Build history of the part. All positions in model axes, mm. Face numbers are marked on the shaded views. A direction names the side the tool comes from. Round coordinates to 2 decimals unless told otherwise and drop trailing zeros. Write each loop counter-clockwise with the first axis right and the second up, starting at its lowest first coordinate (ties: lowest second). Pieces come first, ordered by that corner, then holes. Notation, with made-up numbers: (-40, 86.25) - (16, 86.25) arc R19 cw to (16, 93.25) - close; hole circle Ø6 at (76, -22.75). An arc over 180 degrees is marked (long way). Answer as a JSON object with one key per item and string values. Group by question number.
Item 1: Slice it at D-D, the plane z = 3.25. List the corners of the cut face in (x, y), then the cut area to 3 significant figures.
Item 2: Slice it at B-B, the plane y = 0.75. List the corners of the cut face in (x, z), then the cut area to 3 significant figures.
Item 3: Which spindle directions (+Z, -Z, +X, -X, +Y, -Y) get a long thin tool onto all of the face, cutting with end or side? Do the marked faces 1, 2 and 3. Say none if no direction does.
Item 4: Flat gauge pins, fed straight in: pin 1 (1.2 mm diameter, centred on x = -9.5, z = 7, fed in from -Y); pin 2 (0.6 mm diameter, centred on y = -7.5, z = 4.5, fed in from -X); pin 3 (3 mm diameter, centred on x = 9, z = 4, fed in from +Y); pin 4 (0.5 mm diameter, centred on y = 9, z = 5, fed in from +X). Where does each tip first touch, or does it go through?
Item 5: Probe line 1 (X direction, y = -3.25, z = 5.75); line 2 (Y direction, x = -6, z = 4.25); line 3 (Y direction, x = -8.75, z = 4). List the from-to ranges inside material, lowest first. Write a range as from..to.
Item 6: Slice it at A-A, the plane x = 0. List the corners of the cut face in (y, z).
Item 7: Two-plate mould, pull along Y, no slides. Class the marked faces 4, 5 and 6: +Y half, -Y half, draft (parallel to the pull), parting line (faces both ways), or undercut.
Item 8: Slice it at C-C, the plane x = 5.5. List the corners of the cut face in (y, z).
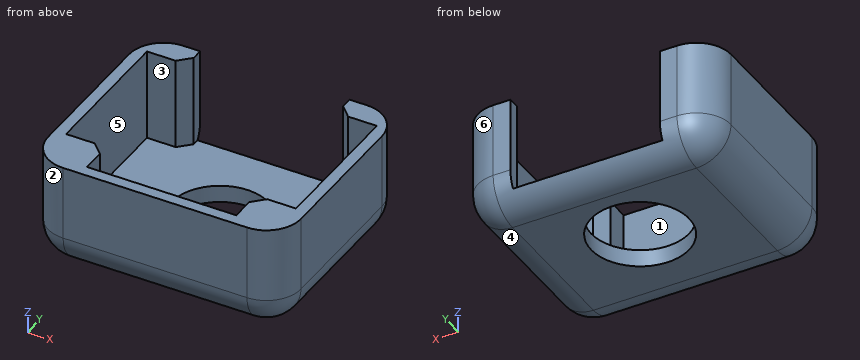
Solid Edge part; units mm, degrees
sketch "Sketch1" plane through (0, 0, 0) normal (0, 0, 1) x (1, 0, 0)
  line L0 (-11, -9.25) -> (11, -9.25)
  line L1 (11, -9.25) -> (11, 9.25)
  line L2 (11, 9.25) -> (-11, 9.25)
  line L3 (-11, 9.25) -> (-11, -9.25)
  circle A0 centre (0, 0.75) radius 4.25
  dimension "D1" = 11
  dimension "D2" = 11
extrude "Protrusion1" add sketch "Sketch1" along normal blind 1.5
sketch "Sketch2" plane through (0, 0, 1.5) normal (0, 0, 1) x (1, 0, 0)
  line L0 (11, -9.25) -> (6, -9.25)
  line L1 (6, -9.25) -> (6, -4.75)
  line L2 (6, -4.75) -> (11, -4.75)
  line L3 (11, -4.75) -> (11, -9.25)
  line L4 (-11, -9.25) -> (-6, -9.25)
  line L5 (-6, -9.25) -> (-6, -4.75)
  line L6 (-6, -4.75) -> (-11, -4.75)
  line L7 (-11, -4.75) -> (-11, -9.25)
  dimension "D1" = 11
  dimension "D2" = 11
  dimension "D3" = 11
  dimension "D4" = 11
extrude "bottom_extension" add sketch "Sketch2" along normal blind 8
sketch "Sketch3" plane through (0, 0, 1.5) normal (0, 0, 1) x (1, 0, 0)
  line L0 (-6, -9.25) -> (6, -9.25)
  line L1 (6, -9.25) -> (6, -8.25)
  line L2 (6, -8.25) -> (-6, -8.25)
  line L3 (-6, -8.25) -> (-6, -9.25)
  dimension "D1" = 6
extrude "Protrusion2" add sketch "Sketch3" along normal up to vertex (8 mm away)
sketch "Sketch4" plane through (0, 0.5, 1.5) normal (0, 0, 1) x (1, 0, 0)
  line L0 (11, 8.75) -> (6, 8.75)
  line L1 (6, 8.75) -> (6, 6.75)
  line L2 (6, 6.75) -> (11, 6.75)
  line L3 (11, 6.75) -> (11, 8.75)
  line L4 (-11, 8.75) -> (-6, 8.75)
  line L5 (-6, 8.75) -> (-6, 6.75)
  line L6 (-6, 6.75) -> (-11, 6.75)
  line L7 (-11, 6.75) -> (-11, 8.75)
  dimension "D1" = 11
  dimension "D2" = 11
extrude "Protrusion3" add sketch "Sketch4" along normal up to vertex (8 mm away)
sketch "Sketch5" plane through (0, 0.5, 1.5) normal (0, 0, 1) x (1, 0, 0)
  line L0 (-11, 6.75) -> (-10, 6.75)
  line L1 (-10, 6.75) -> (-10, -5.25)
  line L2 (-10, -5.25) -> (-11, -5.25)
  line L3 (-11, -5.25) -> (-11, 6.75)
  line L4 (11, -5.25) -> (10, -5.25)
  line L5 (10, -5.25) -> (10, 6.75)
  line L6 (10, 6.75) -> (11, 6.75)
  line L7 (11, 6.75) -> (11, -5.25)
  dimension "D1" = 11
  dimension "D2" = 11
extrude "Protrusion4" add sketch "Sketch5" along normal up to vertex (8 mm away)
fillet "Verrundung_1" radius 3 4 edges at (-11, 9.25, 4.75) (11, 9.25, 4.75) (11, -9.25, 4.75) (-11, -9.25, 4.75)
fillet "Verrundung_2" radius 3 7 edges at (0, -9.25, 0) (10.1213, -8.3713, 0) (11, 0, 0) (0, 9.25, 0) (-10.1213, 8.3713, 0) (-11, 0, 0) (-10.1213, -8.3713, 0)
sketch "Sketch6" plane through (0, 0, 9.5) normal (0, 0, 1) x (1, 0, 0)
  line L0 (-6, 9.25) -> (-6.5, 9.25)
  line L1 (-6.5, 9.25) -> (-6.5, 7.25)
  line L2 (-6.5, 7.25) -> (-6, 7.25)
  line L3 (-6, 7.25) -> (-6, 9.25)
  line L4 (6, 9.25) -> (6.5, 9.25)
  line L5 (6.5, 9.25) -> (6.5, 7.25)
  line L6 (6.5, 7.25) -> (6, 7.25)
  line L7 (6, 7.25) -> (6, 9.25)
  line L8 (-10, -4.75) -> (-6, -4.75)
  line L9 (-6, -4.75) -> (-6, -8.25)
  line L10 (-6.5, -8.25) -> (-6, -8.25)
  line L11 (-6.5, -5.25) -> (-6.5, -8.25)
  line L12 (-10, -5.25) -> (-6.5, -5.25)
  line L13 (-10, -5.25) -> (-10, -4.75)
  line L14 (6, -4.75) -> (10, -4.75)
  line L15 (10, -4.75) -> (10, -5.25)
  line L16 (10, -5.25) -> (6.5, -5.25)
  line L17 (6.5, -5.25) -> (6.5, -8.25)
  line L18 (6.5, -8.25) -> (6, -8.25)
  line L19 (6, -8.25) -> (6, -4.75)
  dimension "D1" = 6
extrude "Cutout1" cut sketch "Sketch6" against normal up to vertex (8 mm away)
chamfer "Fase_2" distance 1 angle 45 4 edges at (-6.5, 7.25, 5.5) (6.5, 7.25, 5.5) (6.5, -5.25, 5.5) (-6.5, -5.25, 5.5)
properties material "ABS-Plastik, mittelfest"
Geometry says:
{
 "1": {"outline": "(-11, -6.25) arc R3 ccw to (-8, -9.25) - (8, -9.25) arc R3 ccw to (11, -6.25) - (11, 6.25) arc R3 ccw to (8, 9.25) - (6.5, 9.25) - (6.5, 8.25) - (7.5, 7.25) - (10, 7.25) - (10, -5.25) - (7.5, -5.25) - (6.5, -6.25) - (6.5, -8.25) - (-6.5, -8.25) - (-6.5, -6.25) - (-7.5, -5.25) - (-10, -5.25) - (-10, 7.25) - (-7.5, 7.25) - (-6.5, 8.25) - (-6.5, 9.25) - (-8, 9.25) arc R3 ccw to (-11, 6.25) - close", "area": "82.3 mm^2"},
 "2": {"outline": "(-11, 3) arc R3 ccw to (-8, 0) - (-4.25, 0) - (-4.25, 1.5) - (-10, 1.5) - (-10, 9.5) - (-11, 9.5) - close; (4.25, 0) - (8, 0) arc R3 ccw to (11, 3) - (11, 9.5) - (10, 9.5) - (10, 1.5) - (4.25, 1.5) - close", "area": "32.4 mm^2"},
 "3": {"face 1": "+Z, +Y", "face 2": "+Z, -Z, -X, -Y", "face 3": "+Z"},
 "4": {"pin 1": "stops at y = -9.11", "pin 2": "stops at x = -10.85", "pin 3": "stops at y = 9.25", "pin 4": "stops at x = 9.66"},
 "5": {"line 1": "x = -11..-10, 10..11", "line 2": "y = -9.25..-8.25", "line 3": "y = -9.15..-5.25, 7.25..9.15"},
 "6": {"outline": "(-9.25, 3) arc R3 ccw to (-6.25, 0) - (-3.5, 0) - (-3.5, 1.5) - (-8.25, 1.5) - (-8.25, 9.5) - (-9.25, 9.5) - close; (5, 0) - (6.25, 0) arc R3 ccw to (8.85, 1.5) - (5, 1.5) - close"},
 "7": {"face 4": "draft", "face 5": "undercut", "face 6": "+Y half"},
 "8": {"outline": "(-9.25, 3) arc R3 ccw to (-6.25, 0) - (6.25, 0) arc R3 ccw to (8.85, 1.5) - (-8.25, 1.5) - (-8.25, 9.5) - (-9.25, 9.5) - close"}
}
